Geometry check sheet. Reference: the model listing, model coordinates, mm. Face numbers are marked on the shaded views. A direction names the side the tool comes from. Give positions to 0.01 mm unless a question says otherwise; leave off trailing zeros. Order: outer loops, then holes, each group sorted by start corner. A loop starts at its lowest first (then second) coordinate and runs counter-clockwise, first axis right, second up. Notation, with made-up numbers: M 34.5,-21 L 67.5,-21 A32 cw 67.5,6 Z; hole C 55,-26.75 d1. An arc over 180 degrees is marked long. Answer as CSV lines item,"result". Start each with the question number.
Q1. Go/stop test with flat-tipped pins: pin 1 (15 mm diameter, centred on x = 25.5, y = -11, fed in from +Z); pin 2 (19.5 mm diameter, centred on x = 47, z = 50, fed in from -Y); pin 3 (5.5 mm diameter, centred on y = -21, z = 2, fed in from -X). Record where each tip stops, or that it passes through.
Q2. Section check D-D, the plane x = 59.5. Record the boundary of the cut face in (y, z).
Q3. Set-up check for the marked faces 4 and 5: record each of +Z, -Z, +X, -X, +Y, -Y from which the full face is reachable in a straight line by a thin tool's end or side.
Q4. Section check A-A, the plane y = 131.5. Record the boundary of the cut face in (x, z), then the cut area to 3 significant figures.
Q5. Thickness scan on line 1 (Y direction, x = 58, z = 98.5); line 2 (Z direction, x = 16, y = 178); line 3 (Z direction, x = 11, y = 91). Record the ranges inside material, lowest first.
Q6. Section check C-C, the plane z = 23.5. Record the boundary of the cut face in (x, y).
Q7. Section check B-B, the plane x = 16.5. Record the boundary of the cut face in (y, z), then the cut area to 3 significant figures.
Q8. Mould release check, pull along Z, two halves, no side actions. Record for the marked faces 1, 2 and 3: +Z half, -Z half, draft (parallel to the pull), parting line (faces both ways), or undercut.
```python
from build123d import *

# Parameters (mm, degrees)
F1_DEPTH = 30
F2_R     = 5.9068086224
F3_DEPTH = 37.3459064877
F5_DEPTH = 254
F6_R     = 5.3482830895
F7_DEPTH = 25.4
F8_DEPTH = 49.7385416959


with BuildPart() as f1:
    # F0 (on Front) → F1 (new body)
    with BuildSketch(Plane.XZ):
        Polygon((0, 5), (0, 0), (41, 0), (41, 56.516070229), (34.2285000014, 91.6807044894), (64.7796728897, 97.563810386), (63.8342146871, 102.4736076107), (28.0746837728, 95.5875509623), (36, 54.4311090238), (36, 5), align=None)
    extrude(amount=F1_DEPTH)

    # F2 (on face) → F3 (cut, through all)
    with BuildSketch(Plane(origin=(44.8195825231, 0, 8.6307112067), x_dir=(0, -1, 0), z_dir=(-0.9819594449, 0, -0.1890916405))):
        with Locations((15.3243150562, 67.6144137979)):
            Circle(F2_R)
    extrude(amount=-F3_DEPTH, mode=Mode.SUBTRACT)

    # F4 (on face) → F5 (join, symmetric)
    with BuildSketch(Plane(origin=(0, 0, 0), x_dir=(-1, 0, 0), z_dir=(0, 1, 0))):
        Polygon((4.1697587408, 89.3783795312), (-28.0746837728, 95.5875509623), (-35.362594468, 57.7411780502), (-3.1181519544, 51.5320066191), align=None)
        Polygon((-31.4480777671, 60.8430350679), (-24.8551371776, 91.4274895161), (0, 86.6412443325), (-5.9146662272, 55.9261775534), align=None, mode=Mode.SUBTRACT)
    extrude(amount=F5_DEPTH, both=True)

    # F6 (on face) → F7 (cut)
    with BuildSketch(Plane(origin=(0, 0, 0), x_dir=(1, 0, 0), z_dir=(0, 0, -1))):
        with Locations((17.5516102463, 14.9040622637)):
            Circle(F6_R)
    extrude(amount=-F7_DEPTH, mode=Mode.SUBTRACT)

    # F8 (cut, through all): a face of the model
    f8_faces = [f1.faces().sort_by_distance(p)[0] for p in [
        (32.0342620964, -15.3243150562, 75.0253234491),
    ]]
    extrude(f8_faces, amount=-F8_DEPTH, mode=Mode.SUBTRACT)


solid = f1.part
```
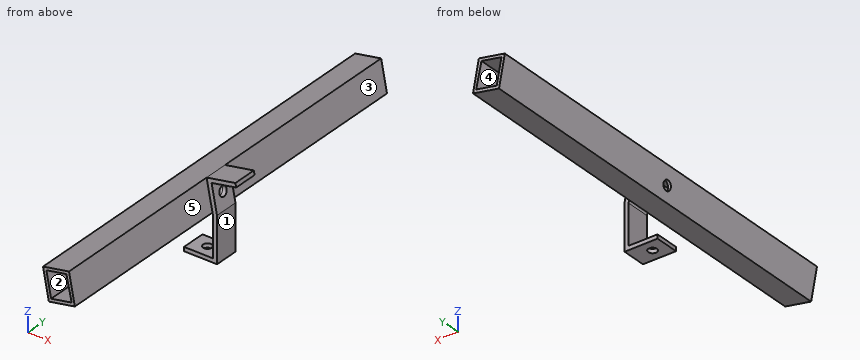
Answer block:
1,pin 1,"stops at z = 96.54"
1,pin 2,"stops at y = -30"
1,pin 3,"stops at x = 0"
2,outline,"M -30,96.55 L 0,96.55 L 0,101.64 L -30,101.64 Z"
3,face 4,"+Y, -Y"
3,face 5,"+Z, +X, -Y"
4,outline,"M -4.17,89.38 L 3.12,51.53 L 35.36,57.74 L 28.07,95.59 Z; hole M 0,86.64 L 5.91,55.93 L 31.45,60.84 L 24.86,91.43 Z"
4,area,"463 mm2"
5,line 1,"y = -30 to 0"
5,line 2,"z = 54.01 to 57.87, 89.72 to 93.26"
5,line 3,"z = 53.05 to 56.91, 88.76 to 92.3"
6,outline,"M 36,-30 L 41,-30 L 41,0 L 36,0 Z"
7,outline,"M -254,54.11 L 254,54.11 L 254,57.96 L -254,57.96 Z; M -254,89.82 L 254,89.82 L 254,93.36 L -254,93.36 Z; M -30,0 L -20.15,0 L -20.15,5 L -30,5 Z; M -9.66,0 L 0,0 L 0,5 L -9.66,5 Z"
7,area,"3,850 mm2"
8,face 1,"draft"
8,face 2,"undercut"
8,face 3,"+Z half"
